```python
from build123d import *

# Parameters (mm, degrees)
F0_W     = 50.8
F0_H     = 50.8
F1_DEPTH = 12.7
F3_DEPTH = 6.35


with BuildPart() as f1:
    # F0 (on Top) → F1 (new body)
    with BuildSketch(Plane.XY):
        with Locations((-25.4, 25.4)):
            Rectangle(F0_W, F0_H)
    extrude(amount=-F1_DEPTH)

    # F2 (on face) → F3 (join)
    with BuildSketch(Plane.XY):
        with BuildLine():
            Line((0, 50.8), (-50.8, 50.8))
            ThreePointArc((-50.8, 50.8), (-25.4, 25.4), (0, 50.8))
        make_face()
    extrude(amount=F3_DEPTH)


solid = f1.part
```
For this review, take the finished solid that the model builds, in its own axes (mm). A direction names the side the tool comes from. Round coordinates to 2 decimals unless told otherwise and drop trailing zeros. Write each loop counter-clockwise with the first axis right and the second up, starting at its lowest first coordinate (ties: lowest second). Pieces come first, ordered by that corner, then holes. Notation, with made-up numbers: (78, 80) -> (112, 80) arc R16 ccw to (112, 104) -> close; hole circle Ø1 at (52, 43). An arc over 180 degrees is marked (long way). One line per question, with ' | ' between items. Start each with the question number.
(1) Add section D-D, the plane y = 38. Write out the cut boundary in (x, z).
(2) Insertion check: P1, Ø1.5, axis at y = 41.5, z = 2, coming from the +X side; P2, Ø2, axis at x = -22.5, y = 16.5, coming from the +Z side. Each pin has a flat end and moves straight along its axis. Give the tip position at first contact, or say it passes through.
(3) Add section A-A, the plane y = 17.5. Write out the cut boundary in (x, z).
(4) Tool access review of faces 1 (the face through (-26, 14, 0)), 2 (the face through (-26, 41, 6.35)): name each direction out of +Z, -Z, +X, -X, +Y, -Y from which nothing blocks a thin tool from reaching the whole face with its end or side.
(5) For line 1 along Z through (x, y) = (-24, 15); line 2 along Y through (x, z) = (-16.5, 5); line 3 along Y through (x, z) = (-7, 5.5), list the stretches that pass through material, from the lowest coordinate up. Write a range as from..to.
(6) Add section C-C, the plane z = 5. Write out the cut boundary in (x, y).
(7) Add section B-B, the plane x = -25.4. Write out the cut boundary in (y, z).
Answer list:
1) outline: (-50.8, -12.7) -> (0, -12.7) -> (0, 0) -> (-3.46, 0) -> (-3.46, 6.35) -> (-47.34, 6.35) -> (-47.34, 0) -> (-50.8, 0) -> close
2) P1: x = -1.48 | P2: z = 0
3) outline: (-50.8, -12.7) -> (0, -12.7) -> (0, 0) -> (-50.8, 0) -> close
4) face 1: +Z, -Y | face 2: +Z, +X, -X, +Y, -Y
5) line 1: -12.7..0 | line 2: 27.01..50.8 | line 3: 33.29..50.8
6) outline: (-50.8, 50.8) arc R25.4 ccw to (0, 50.8) -> close
7) outline: (0, -12.7) -> (50.8, -12.7) -> (50.8, 6.35) -> (25.4, 6.35) -> (25.4, 0) -> (0, 0) -> close
